```python
from build123d import *

# Parameters (mm, degrees)
SKETCH1_R           = 25
SKETCH1_R_2         = 18
SKETCH1_R_3         = 1
BOSS_EXTRUDE2_DEPTH = 1.6
SKETCH2_W           = 1.2
SKETCH2_H           = 2.3
BOSS_EXTRUDE3_DEPTH = 0.1


with BuildPart() as part:
    # Sketch1 → Boss-Extrude2 (new body)
    with BuildSketch(Plane.XY):
        Circle(SKETCH1_R)
        Circle(SKETCH1_R_2, mode=Mode.SUBTRACT)
        with Locations((16.086679272, -16.086679272)):
            Circle(SKETCH1_R_3, mode=Mode.SUBTRACT)
        with Locations((-16.086679272, -16.086679272)):
            Circle(SKETCH1_R_3, mode=Mode.SUBTRACT)
        with Locations((-16.086679272, 16.086679272)):
            Circle(SKETCH1_R_3, mode=Mode.SUBTRACT)
        with Locations((16.086679272, 16.086679272)):
            Circle(SKETCH1_R_3, mode=Mode.SUBTRACT)
    extrude(amount=BOSS_EXTRUDE2_DEPTH)

    # Sketch2 → Boss-Extrude3 (add)
    with BuildSketch(Plane.XY):
        with Locations((1.3, 22.65)):
            Rectangle(SKETCH2_W, SKETCH2_H)
        with Locations((3.9, 22.65)):
            Rectangle(SKETCH2_W, SKETCH2_H)
        with Locations((-3.9, 22.65)):
            Rectangle(SKETCH2_W, SKETCH2_H)
        with Locations((-1.3, 22.65)):
            Rectangle(SKETCH2_W, SKETCH2_H)
    extrude(amount=-BOSS_EXTRUDE3_DEPTH)


solid = part.part
```
Model file for the job. Use its own axes, mm. Coordinates: 2 decimals unless noted, no trailing zeros. Loops run counter-clockwise (first coordinate to the right, second up) from the corner with the lowest first, then second, coordinate; pieces in that order, holes last. Notation, with made-up numbers: (50, 30.5) - (99, 30.5) arc R18 cw to (99, 48.5) - close; hole circle Ø2 at (41.5, -7.5). An arc over 180 degrees is marked (long way). Write item = value, one per line. Start each with the question number.
Item 1: Saw through at C-C, the plane z = 0.5. List the corners of the cut face in (x, y).
Item 2: Drop flat-ended pins along their axis: pin 1 Ø1 at (x, y) = (13.5, -14.5) entering from -Z; pin 2 Ø1.2 at (x, y) = (-16.09, -16.09) entering from -Z. Give the stop position or say it passes through.
Item 3: Saw through at A-A, the plane x = 0. List the corners of the cut face in (y, z).
Item 4: Pull direction X, two halves, no side cores. Call faces 1 (the face through (-4, 23, -0.1)), 2 (the face through (23.846, 7.509, 0.789)), 3 (the face through (-16.824, -15.411, 0.789)): +X half, -X half, draft (parallel to the pull), parting line (faces both ways), or undercut.
Item 5: Wall check: probe 1 along Y at (x, z) = (-16, 0.55); probe 2 along Y at (x, z) = (0, 0.9); probe 3 along Z at (x, y) = (-13, -16). Give the ranges that are in metal, low to high. Write a range as [from, to].
Item 6: Saw through at D-D, the plane y = 20. List the corners of the cut face in (x, z), then the cut area to 3 significant figures.
Answers:
q1.outline = circle Ø50 at (0, 0); hole circle Ø36 at (0, 0); hole circle Ø2 at (-16.09, -16.09); hole circle Ø2 at (-16.09, 16.09); hole circle Ø2 at (16.09, -16.09); hole circle Ø2 at (16.09, 16.09)
q2.pin_1 = 0
q2.pin_2 = through
q3.outline = (-25, 0) - (-18, 0) - (-18, 1.6) - (-25, 1.6) - close; (18, 0) - (25, 0) - (25, 1.6) - (18, 1.6) - close
q4.face_1 = draft
q4.face_2 = parting line
q4.face_3 = undercut
q5.probe_1 = [-19.21, -17.08], [-15.09, -8.25], [8.25, 15.09], [17.08, 19.21]
q5.probe_2 = [-25, -18], [18, 25]
q5.probe_3 = [0, 1.6]
q6.outline = (-15, 0) - (15, 0) - (15, 1.6) - (-15, 1.6) - close
q6.area = 48.0 mm2
